Work out the finished part from the listing and answer in its coordinate system (mm). Face numbers are marked on the shaded views. Round coordinates to 2 decimals unless told otherwise and drop trailing zeros. Write each loop counter-clockwise with the first axis right and the second up, starting at its lowest first coordinate (ties: lowest second). Pieces come first, ordered by that corner, then holes.
1. Find section C-C (x = 22). Write down the section's boundary in (y, z), and give its area (3 significant figures).
2. Flat-ended cylindrical pins translate along their axes: pin 1 Ø4 at (x, z) = (14, 4.5) entering from -Y; pin 2 Ø1 at (x, y) = (44.5, 9) entering from -Z; pin 3 Ø2 at (x, y) = (41, 9) entering from -Z. Find the tip coordinate at first contact, or state that the pin passes through.
3. Find section A-A (z = 0). Write down the section's boundary in (x, y), and give its area (3 significant figures).
4. Find section B-B (x = 6). Write down the section's boundary in (y, z).
5. Determine the mould class of the marked faces 1, 2 and 3 for opening direction Y: pulls with the +Y half, pulls with the -Y half, needs draft (parallel to the pull), parting line crosses it, or undercut.
6. Straight lines are drawn through the part: probe 1 along Y at (x, z) = (34, -0.25); probe 2 along Y at (x, z) = (3.5, -3.75); probe 3 along Y at (x, z) = (45.5, -5.25). For each, find the intervals that lie inside material, in ascending order.
```python
from build123d import *

# Parameters (mm, degrees)
HEX_2_DEPTH = 15


with BuildPart() as part:
    # BodySke → BaseBody (revolve)
    with BuildSketch(Plane.XY, mode=Mode.PRIVATE) as basebody_sk:
        with BuildLine():
            Line((0, 0), (0, 10.352))
            Line((0, 10.352), (0.951473244, 12))
            Line((0.951473244, 12), (47.811947441, 12))
            ThreePointArc((47.811947441, 12), (49.448514264, 6.098925602), (50, 0))
            Line((50, 0), (0, 0))
        make_face()
    revolve(basebody_sk.sketch.rotate(Axis((-12.7, 0, 0), (1, 0, 0)), 90), axis=Axis((-12.7, 0, 0), (1, 0, 0)))

    # Sketch2 → Hex 2 (cut)
    with BuildSketch(Plane.ZY):
        Polygon((3.464101615, 6), (-3.464101615, 6), (-6.92820323, 0), (-3.464101615, -6), (3.464101615, -6), (6.92820323, 0), align=None)
    extrude(amount=-HEX_2_DEPTH, mode=Mode.SUBTRACT)


solid = part.part
```
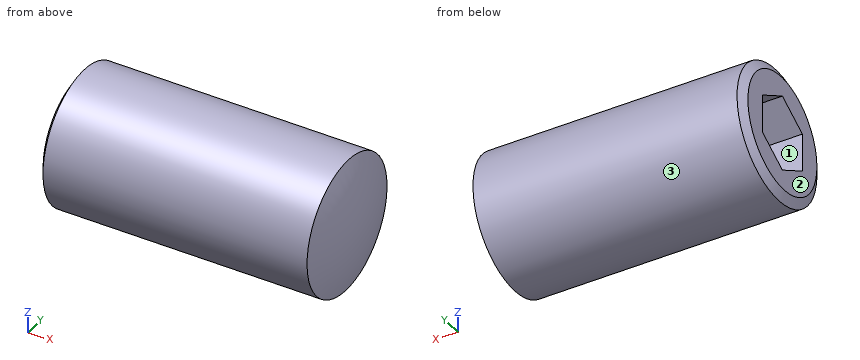
Worked answers:
1. outline: circle Ø24 at (0, 0)
1. area: 452 mm2
2. pin 1: stops at y = -11.74
2. pin 2: stops at z = -8.47
2. pin 3: stops at z = -8.94
3. outline: (0, -10.35) - (0.95, -12) - (47.81, -12) arc R34 ccw to (47.81, 12) - (0.95, 12) - (0, 10.35) - (0, 6) - (15, 6) - (15, -6) - (0, -6) - close
3. area: 1,000 mm2
4. outline: circle Ø24 at (0, 0); hole (-6, -3.46) - (0, -6.93) - (6, -3.46) - (6, 3.46) - (0, 6.93) - (-6, 3.46) - close
5. face 1: undercut
5. face 2: needs draft
5. face 3: parting line crosses it
6. probe 1: y = -12 to 12
6. probe 2: y = -11.4 to -5.5, 5.5 to 11.4
6. probe 3: y = -10.79 to 10.79
